from build123d import *

# Parameters (mm, degrees)
BOSS_EXTRUDE1_DEPTH = 4.699
SKETCH2_R           = 1.905
SKETCH2_R_2         = 2.032
SKETCH2_W           = 40.259
SKETCH2_H           = 20.0152
CUT_EXTRUDE1_DEPTH  = 105.14657371
FILLET1_R           = 1.27


with BuildPart() as part:
    # Sketch1 → Boss-Extrude1 (new body)
    with BuildSketch(Plane(origin=(0, 0, 0), x_dir=(1, 0, 0), z_dir=(0, 1, 0))):
        with BuildLine():
            Line((-20.1295, 14.5796), (29.0195, 14.5796))
            add(Edge.make_bspline(
                [(29.0195, 14.5796), (61.676259281, 14.5796), (92.626496887, 5.406179728), (100.540261174, 3.042166683)],
                knots=[0, 0, 0, 0, 1, 1, 1, 1], degree=3))
            ThreePointArc((100.540261174, 3.042166683), (102.777881706, -0.425331821), (99.699916451, -3.174262779))
            add(Edge.make_bspline(
                [(29.0195, -15.9766), (36.752411566, -15.9766), (47.448783559, -11.662139755), (61.563248496, -6.964298313), (74.754433056, -4.344440996), (91.245915547, -3.356476028), (99.699916451, -3.174262779)],
                knots=[0, 0, 0, 0, 0.316402814, 0.381996868, 0.65594054, 1, 1, 1, 1], degree=3))
            Line((29.0195, -15.9766), (-20.1295, -15.9766))
            add(Edge.make_bspline(
                [(-20.1295, 14.5796), (-25.650459674, 14.5796), (-34.705495366, -0.225155417), (-29.383489197, -15.9766), (-20.1295, -15.9766)],
                knots=[0, 0, 0, 0, 0.484878873, 1, 1, 1, 1], degree=3))
        make_face()
    extrude(amount=BOSS_EXTRUDE1_DEPTH)

    # Sketch2 → Cut-Extrude1 (cut, through all)
    with BuildSketch(Plane(origin=(0, 4.699, 0), x_dir=(1, 0, 0), z_dir=(0, 1, 0))):
        with Locations((62.4205, 2.803132377)):
            Circle(SKETCH2_R)
        with Locations(Location((-24.71166, 4.92506, 0), (0, 0, 270))):
            Circle(SKETCH2_R_2)
        with Locations(Location((-24.71166, -4.92506, 0), (0, 0, 270))):
            Circle(SKETCH2_R_2)
        with Locations(Location((24.71166, -4.92506, 0), (0, 0, 270))):
            Circle(SKETCH2_R_2)
        with Locations(Location((24.71166, 4.92506, 0), (0, 0, 270))):
            Circle(SKETCH2_R_2)
        with BuildLine():
            Line((29.0195, 0), (29.0195, 8.262060115))
            add(Edge.make_bspline(
                [(29.0195, 8.262060115), (49.82184103, 7.331297412), (62.803182548, 4.669299323)],
                knots=[0, 0, 0, 1, 1, 1], degree=2))
            ThreePointArc((62.803182548, 4.669299323), (64.32549921, 2.801397362), (62.799782619, 0.936271457))
            add(Edge.make_bspline(
                [(62.799782619, 0.936271457), (48.06851018, -2.056621868), (29.0195, -9.517939885)],
                knots=[0, 0, 0, 1, 1, 1], degree=2))
            Line((29.0195, -9.517939885), (29.0195, 0))
        make_face()
        Rectangle(SKETCH2_W, SKETCH2_H)
    extrude(amount=-CUT_EXTRUDE1_DEPTH, mode=Mode.SUBTRACT)

    # Fillet1
    fillet1_edges = [part.edges().sort_by_distance(p)[0] for p in [
        (29.0195, 2.3495, 9.517939885),
        (29.0195, 2.3495, -8.262060115),
    ]]
    fillet(fillet1_edges, radius=FILLET1_R)


solid = part.part
Geometry check sheet. Reference: the model listing, model coordinates, mm. A direction names the side the tool comes from. Give positions to 0.01 mm unless a question says otherwise; leave off trailing zeros. Write each question's results on one line, items separated by ' | '.
1) Release check for a two-part mould opening along Z. For faces 3 (the face through (22.73, 2.38, -5.37)), 4 (the face through (5, 2, 15.977)), 5 (the face through (35, 0, 11)) record: +Z half, -Z half, draft (parallel to the pull), parting line (faces both ways), or undercut.
Answers follow:
face 3: undercut | face 4: +Z half | face 5: draft
2) Thickness scan on line 1 (Z direction, x = -1, y = 3.65); line 2 (Z direction, x = 32, y = 4.35); line 3 (Z direction, x = 87.5, y = 2.85). Record the ranges inside material, lowest first.
Answers follow:
line 1: -14.58 to -10.01, 10.01 to 15.98 | line 2: -14.55 to -8.12, 8.37 to 15.81 | line 3: -6.65 to 3.68
3) Tool access check on faces 1 (the face through (0, 2, 10.008)), 2 (the face through (4, 2, -14.58)). Record the directions out of +Z, -Z, +X, -X, +Y, -Y that give a thin tool (end or side, any length) a straight path to the whole face; none if there is none.
Answers follow:
face 1: +Y, -Y | face 2: -Z, +X, -X, +Y, -Y
4) Gauge pin test, flat ends, axial feed: pin 1 (3.5 mm diameter, centred on x = -24.71, z = 4.93, fed in from -Y); pin 2 (2.5 mm diameter, centred on y = 1.5, z = 5, fed in from -X); pin 3 (2.5 mm diameter, centred on y = 2, z = 1.5, fed in from +X); pin 4 (1 mm diameter, centred on x = 37, y = 2.5, fed in from -Z). Record the tip position at first contact, or that the pin passes through.
Answers follow:
pin 1: through | pin 2: x = -31.26 | pin 3: x = 102.8 | pin 4: z = -14.42
5) Section check A-A, the plane y = 1.05. Count the separate pieces of the cut face and the enclosed holes in it, plus the area to 3 significant figures.
Answers follow:
separate pieces: 1 | enclosed holes: 6 | area: 1,890 mm2
